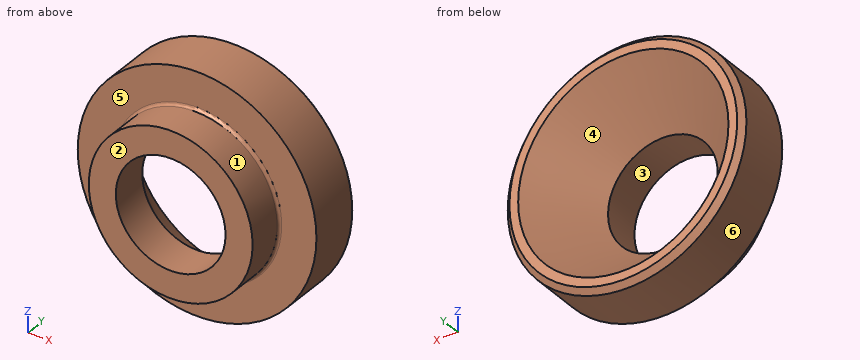
```python
from build123d import *

# Parameters (mm, degrees)
CHAMFER1_SIZE = 0.254
FILLET1_R     = 0.127


with BuildPart() as part:
    # Sketch1 → Revolve1 (revolve)
    with BuildSketch(Plane.XY):
        Polygon((2.5527, 0), (2.5527, 1.778), (4.8895, 4.445), (5.5499, 4.445), (5.5499, 1.778), (3.81, 1.778), (3.81, 0), align=None)
    revolve(axis=Axis((0, 0, 0), (0, 1, 0)))

    # Chamfer1
    chamfer1_edges = [part.edges().sort_by_distance(p)[0] for p in [
        (-5.5499, 4.445, 0),
    ]]
    chamfer(chamfer1_edges, length=CHAMFER1_SIZE)

    # Fillet1
    fillet1_edges = [part.edges().sort_by_distance(p)[0] for p in [
        (-3.81, 1.778, 0),
    ]]
    fillet(fillet1_edges, radius=FILLET1_R)


solid = part.part
```
Part model, mm, in its own coordinate system. Face numbers are marked on the shaded views. A direction names the side the tool comes from. Give positions to 0.01 mm unless a question says otherwise; leave off trailing zeros. Write each loop counter-clockwise with the first axis right and the second up, starting at its lowest first coordinate (ties: lowest second). Pieces come first, ordered by that corner, then holes. Notation, with made-up numbers: (30.25, 89.25) -> (82.25, 89.25) arc R31 ccw to (82.25, 128.25) -> close; hole circle Ø1 at (16, 67). An arc over 180 degrees is marked (long way). Put each result on its own line as item: value. Start each with the question number.
Item 1: Pull direction X, two halves, no side cores. Call the marked faces 3, 4, 5 and 6: pulls with the +X half, pulls with the -X half, needs draft (parallel to the pull), parting line crosses it, or undercut.
Item 2: Wall check: L1, parallel to X at y = 1.25, z = 0; L2, parallel to X at y = 2.5, z = -2. Give the ranges that are in metal, low to high. Write a range as [from, to].
Item 3: Which spindle directions (+Z, -Z, +X, -X, +Y, -Y) get a long thin tool onto all of the face, cutting with end or side? Do the marked faces 1 and 2. Say none if no direction does.
Item 4: Cut at D-D (y = 3.6). List the corners of the cut face in (x, z).
Item 5: Cut at C-C (y = 2.6). List the corners of the cut face in (x, z), then the cut area to 3 significant figures.
Item 6: Pin check, flat tips, straight feed: pin 1 Ø1 at (y, z) = (1, -3) entering from -X; pin 2 Ø1 at (y, z) = (3.5, -2.5) entering from +X; pin 3 Ø6.5 at (x, z) = (0, 0) entering from +Y. Stop position of each tip, or through.
Answer list:
1. face 3: undercut
1. face 4: undercut
1. face 5: needs draft
1. face 6: parting line crosses it
2. L1: x = [-3.81, -2.55], [2.55, 3.81]
2. L2: x = [-5.18, -2.48], [2.48, 5.18]
3. face 1: -Y
3. face 2: +Z, -Z, +X, -X, -Y
4. outline: circle Ø11.1 at (0, 0); hole circle Ø8.3 at (0, 0)
5. outline: circle Ø11.1 at (0, 0); hole circle Ø6.55 at (0, 0)
5. area: 63.1 mm2
6. pin 1: stops at x = -2.88
6. pin 2: stops at x = 5.18
6. pin 3: stops at y = 2.57
